```python
from build123d import *

# Parameters (mm, degrees)
SKETCH1_W           = 75
SKETCH1_H           = 25
BOSS_EXTRUDE1_DEPTH = 1
SKETCH3_W           = 75
SKETCH3_H           = 24
BOSS_EXTRUDE2_DEPTH = 1
SKETCH4_W           = 75
SKETCH4_H           = 12
SKETCH4_R           = 2
BOSS_EXTRUDE3_DEPTH = 1
FILLET1_R           = 4
CUT_EXTRUDE2_REACH  = 62.869
SKETCH6_R           = 4.25
FILLET2_R           = 5


with BuildPart() as part:
    # Sketch1 → Boss-Extrude1 (new body)
    with BuildSketch(Plane(origin=(0, 0, 0), x_dir=(1, 0, 0), z_dir=(0, 1, 0))):
        with Locations((-12.5, -2.5)):
            Rectangle(SKETCH1_W, SKETCH1_H)
    extrude(amount=BOSS_EXTRUDE1_DEPTH)

    # Sketch3 → Boss-Extrude2 (add)
    with BuildSketch(Plane.XY.offset(15)):
        with Locations((-12.5, -11)):
            Rectangle(SKETCH3_W, SKETCH3_H)
    extrude(amount=BOSS_EXTRUDE2_DEPTH)

    # Sketch4 → Boss-Extrude3 (add)
    with BuildSketch(Plane.XZ.offset(23)):
        with Locations((-12.5, 22)):
            Rectangle(SKETCH4_W, SKETCH4_H)
        with Locations(Location((20.805858618, 24, 0), (0, 0, 270))):
            Circle(SKETCH4_R, mode=Mode.SUBTRACT)
        with Locations(Location((-46, 24, 0), (0, 0, 270))):
            Circle(SKETCH4_R, mode=Mode.SUBTRACT)
    extrude(amount=-BOSS_EXTRUDE3_DEPTH)

    # Fillet1
    fillet1_edges = [part.edges().sort_by_distance(p)[0] for p in [
        (-50, -22.5, 28),
        (25, -22.5, 28),
    ]]
    fillet(fillet1_edges, radius=FILLET1_R)

    # Sketch6 → Cut-Extrude2 (cut, up to next)
    with BuildSketch(Plane.XY.offset(16), mode=Mode.PRIVATE) as cut_extrude2_sk1:
        with Locations((-37.172974346, -12)):
            Circle(SKETCH6_R)
    cut_extrude2_tool1 = extrude(cut_extrude2_sk1.sketch, amount=-CUT_EXTRUDE2_REACH, mode=Mode.PRIVATE) & part.part
    # Sketch6 → Cut-Extrude2 (cut, up to next)
    with BuildSketch(Plane.XY.offset(16), mode=Mode.PRIVATE) as cut_extrude2_sk2:
        with Locations((-12.026924054, -12)):
            Circle(SKETCH6_R)
    cut_extrude2_tool2 = extrude(cut_extrude2_sk2.sketch, amount=-CUT_EXTRUDE2_REACH, mode=Mode.PRIVATE) & part.part
    # Sketch6 → Cut-Extrude2 (cut, up to next)
    with BuildSketch(Plane.XY.offset(16), mode=Mode.PRIVATE) as cut_extrude2_sk3:
        with Locations((12.738125476, -12)):
            Circle(SKETCH6_R)
    cut_extrude2_tool3 = extrude(cut_extrude2_sk3.sketch, amount=-CUT_EXTRUDE2_REACH, mode=Mode.PRIVATE) & part.part
    add(cut_extrude2_tool1.solids().sort_by_distance((-37.172974, -12, 16))[0], mode=Mode.SUBTRACT)
    add(cut_extrude2_tool2.solids().sort_by_distance((-12.026924, -12, 16))[0], mode=Mode.SUBTRACT)
    add(cut_extrude2_tool3.solids().sort_by_distance((12.738125, -12, 16))[0], mode=Mode.SUBTRACT)

    # Fillet2
    fillet2_edges = [part.edges().sort_by_distance(p)[0] for p in [
        (-50, 0.5, -10),
        (25, 0.5, -10),
    ]]
    fillet(fillet2_edges, radius=FILLET2_R)


solid = part.part
```
Here's how the part is built. I have some questions about the finished solid (model axes, mm). A direction names the side the tool comes from. Give positions to 0.01 mm unless a question says otherwise; leave off trailing zeros. Loops run counter-clockwise (first coordinate to the right, second up) from the corner with the lowest first, then second, coordinate; pieces in that order, holes last. Notation, with made-up numbers: M -10.75,8.5 L 10.25,8.5 A23 ccw 10.25,29.5 Z; hole C 75.25,16 d10. An arc over 180 degrees is marked long. Use one line per item in the form item = value. Start each with the question number.
Q1. If we section it at D-D (z = 12): Write out the boundary of the cut face in (x, y), then the cut area to 3 significant figures.
Q2. If we section it at C-C (x = -19.5): Write out the boundary of the cut face in (y, z).
Q3. Thinking about a two-plate mould opening in X: for faces 4 (the cylindrical face through (9.37, -14.59, 15.51)), 5 (the flat face through (-13, -16.5, 15)), 6 (the cylindrical face through (-8.1, -13.63, 15.51)), 7 (the cylindrical face through (23.5, 0.51, -8.57)), which applies, +X half, -X half, draft (parallel to the pull), parting line (faces both ways), or undercut?
Q4. Will these pins go through, and if not, where does the flat tip stop? pin 1 Ø6 at (x, y) = (-38.5, -13.5) entering from -Z; pin 2 Ø12.5 at (x, z) = (-3.5, -2.5) entering from -Y; pin 3 Ø11.5 at (x, y) = (-10.5, -11) entering from +Z.
Q5. If we section it at B-B (x = -36): Write out the boundary of the cut face in (y, z).
Q6. I need wall thicknesses on line 1 along X through (y, z) = (-22.7, 24); line 2 along Y through (x, z) = (9, -6.5); line 3 along Z through (x, y) = (-46, -17). Which ranges of each line are inside material? Lowest first, please.
Q7. If we section it at A-A (y = -12): Write out the boundary of the cut face in (x, z).
Q8. Which directions (+Z, -Z, +X, -X, +Y, -Y) give clear straight access to the entire face, cutting with the end or side of a thin tool? Please do faces 1 (the flat face through (-13, -5, 16)), 2 (the cylindrical face through (-48.57, 0.51, -8.5)), 3 (the flat face through (-13, 0, 2)).
Taken from the geometry:
q1.outline = M -50,0 L 25,0 L 25,1 L -50,1 Z
q1.area = 75.0 mm^2
q2.outline = M -23,15 L 0,15 L 0,-10 L 1,-10 L 1,16 L -22,16 L -22,28 L -23,28 Z
q3.face_4 = undercut
q3.face_5 = draft
q3.face_6 = undercut
q3.face_7 = +X half
q4.pin_1 = 15
q4.pin_2 = 0
q4.pin_3 = 16
q5.outline = M -23,15 L -16.08,15 L -16.08,16 L -22,16 L -22,28 L -23,28 Z; M -7.92,15 L 0,15 L 0,-10 L 1,-10 L 1,16 L -7.92,16 Z
q6.line_1 = -50 to -48, -44 to 18.81, 22.81 to 25
q6.line_2 = 0 to 1
q6.line_3 = 15 to 16
q7.outline = M -50,15 L -41.42,15 L -41.42,16 L -50,16 Z; M -32.92,15 L -16.28,15 L -16.28,16 L -32.92,16 Z; M -7.78,15 L 8.49,15 L 8.49,16 L -7.78,16 Z; M 16.99,15 L 25,15 L 25,16 L 16.99,16 Z
q8.face_1 = +Z, +X, -X, +Y
q8.face_2 = -Z, -X, +Y, -Y
q8.face_3 = -Z, +X, -X, -Y
